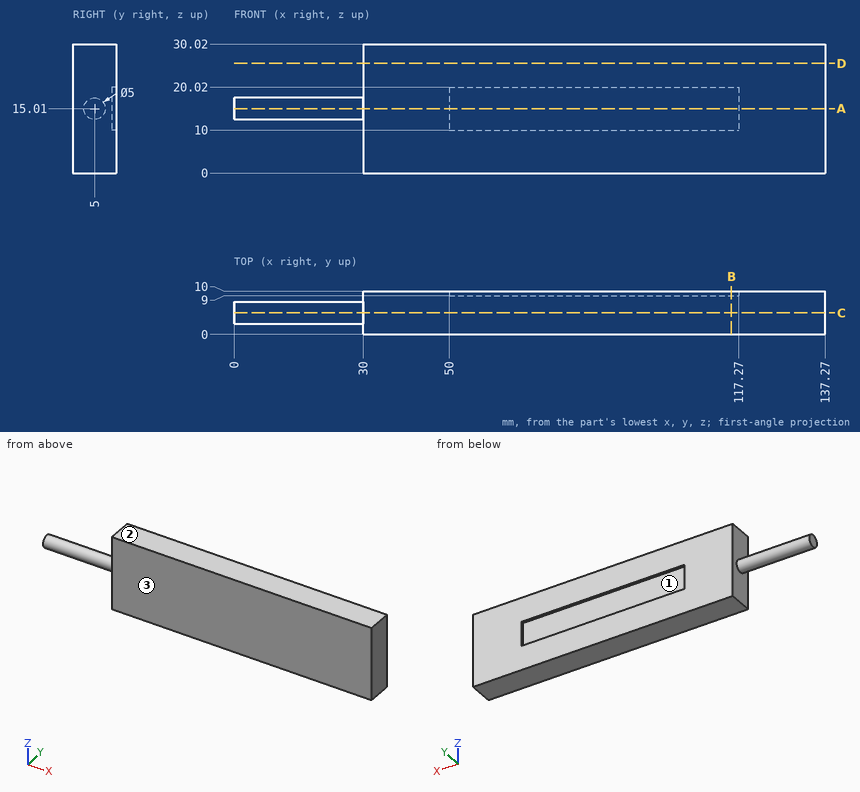
Study the drawing (mm; zero at the part's minimum x, y, z) and answer. Round coordinates to 2 decimals unless told otherwise and drop trailing zeros. Write each loop counter-clockwise with the first axis right and the second up, starting at its lowest first coordinate (ties: lowest second). Pieces come first, ordered by that corner, then holes. Notation, with made-up numbers: (84, 9) -> (103, 9) arc R21 cw to (103, 48) -> close; hole circle Ø2 at (18, 35). An arc over 180 degrees is marked (long way). Answer as CSV lines item,"result". Start each with the question number.
(1) The mould has two halves that part along Z. Classify the marked faces 1, 2 and 3: +Z half, -Z half, draft (parallel to the pull), parting line (faces both ways), or undercut.
(2) The part is cut by section D-D, the plane z = 25.5. Give the vertices of the cut face in (x, y), then the cut area to 3 significant figures.
(3) Each of these flat-tipped pins is pushed along its axis until it touches: pin 1 (3 mm diameter, centred on x = 29.5, z = 21.5, fed in from +Y); pin 2 (2 mm diameter, centred on y = 6.5, z = 19.5, fed in from -X); pin 3 (3 mm diameter, centred on x = 17.5, y = 5, fed in from +Z). Where does it stop, or does it pass through?
(4) Find the intervals of material crossed by probe 1 along X at (y, z) = (4, 12.5); probe 2 along Y at (x, z) = (112.5, 15.5); probe 3 along Y at (x, z) = (21, 13), in increasing order.
(5) The part is cut by section B-B, the plane x = 115.5. Give the vertices of the cut face in (y, z).
(6) The part is cut by section C-C, the plane y = 5. Give the vertices of the cut face in (x, z).
(7) The part is cut by section A-A, the plane z = 15.01. Give the vertices of the cut face in (x, y), then the cut area to 3 significant figures.
Output values:
1,face 1,"undercut"
1,face 2,"+Z half"
1,face 3,"draft"
2,outline,"(30, 0) -> (137.27, 0) -> (137.27, 10) -> (30, 10) -> close"
2,area,"1,070 mm²"
3,pin 1,"stops at y = 10"
3,pin 2,"stops at x = 30"
3,pin 3,"stops at z = 17.51"
4,probe 1,"x = 30 to 137.27"
4,probe 2,"y = 0 to 9"
4,probe 3,"y = 3.51 to 6.49"
5,outline,"(0, 0) -> (10, 0) -> (10, 10) -> (9, 10) -> (9, 20.02) -> (10, 20.02) -> (10, 30.02) -> (0, 30.02) -> close"
6,outline,"(0, 12.51) -> (30, 12.51) -> (30, 0) -> (137.27, 0) -> (137.27, 30.02) -> (30, 30.02) -> (30, 17.51) -> (0, 17.51) -> close"
7,outline,"(0, 2.5) -> (30, 2.5) -> (30, 0) -> (137.27, 0) -> (137.27, 10) -> (117.27, 10) -> (117.27, 9) -> (50, 9) -> (50, 10) -> (30, 10) -> (30, 7.5) -> (0, 7.5) -> close"
7,area,"1,160 mm²"
